from build123d import *

# Parameters (mm, degrees)
SKETCH1_W                      = 7
SKETCH1_H                      = 26.5
SKETCH2_R                      = 12.5
SHAFT_THRU_DEPTH               = 52.39066063
CBORE_FOR_M5_SHCS1_D           = 5.5
CBORE_FOR_M5_SHCS1_CBORE_D     = 10
CBORE_FOR_M5_SHCS1_CBORE_DEPTH = 5
CIRPATTERN1_COUNT              = 4
SKETCH5_R                      = 14.25
SEAL_SEAT_DEPTH                = 3.9624


with BuildPart() as part:
    # Sketch1 → Main_body (revolve)
    with BuildSketch(Plane(origin=(0, 0, 0), x_dir=(0, 0, -1), z_dir=(1, 0, 0)), mode=Mode.PRIVATE) as main_body_sk:
        with Locations((-139.159, -22.75)):
            Rectangle(SKETCH1_W, SKETCH1_H)
        with Locations((-139.159, 22.75)):
            Rectangle(SKETCH1_W, SKETCH1_H)
    revolve(main_body_sk.sketch.rotate(Axis((0, 0, 1000), (0, 0, -1)), 270), axis=Axis((0, 0, 1000), (0, 0, -1)))

    # Sketch2 → Shaft_thru (cut, through all)
    with BuildSketch(Plane(origin=(0, 0, 135.659), x_dir=(-1, 0, 0), z_dir=(0, 0, -1))):
        Circle(SKETCH2_R)
    extrude(amount=-SHAFT_THRU_DEPTH, mode=Mode.SUBTRACT)

    # CBORE for M5 SHCS1 (through all)
    with Locations(Plane.XY.offset(142.659)):
        with Locations((0, 29.3156)):
            cbore_for_m5_shcs1 = CounterBoreHole(CBORE_FOR_M5_SHCS1_D / 2, CBORE_FOR_M5_SHCS1_CBORE_D / 2, CBORE_FOR_M5_SHCS1_CBORE_DEPTH)

    # CirPattern1: CBORE for M5 SHCS1 ×4 about axis
    cirpattern1_axis = Axis((0, 0, 0), (0, 0, 1))
    for i in range(1, CIRPATTERN1_COUNT):
        add(cbore_for_m5_shcs1.rotate(cirpattern1_axis, i * 360 / CIRPATTERN1_COUNT), mode=Mode.SUBTRACT)

    # Sketch5 → seal_seat (cut)
    with BuildSketch(Plane.XY.offset(142.659)):
        Circle(SKETCH5_R)
    extrude(amount=-SEAL_SEAT_DEPTH, mode=Mode.SUBTRACT)


solid = part.part
Geometry: final body of the model. Coordinates: model frame, mm. A direction names the side the tool comes from. Coordinates: 2 decimals unless noted, no trailing zeros. Order: outer loops, then holes, each group sorted by start corner. A loop starts at its lowest first (then second) coordinate and runs counter-clockwise, first axis right, second up.
(1) Draft query along Y for faces 3 (the face through (-34.34, 10.81, 139.11)), 4 (the face through (0.6, 26.63, 136.64)), 5 (the face through (-1, -15, 142.659)), 6 (the face through (-27, 2, 137.659)). Return one class per face: pulls with the +Y half, pulls with the -Y half, needs draft (parallel to the pull), parting line crosses it, or undercut.
(2) Material intervals for probe 1 along Y at (x, z) = (0, 141.4); probe 2 along Y at (x, z) = (0, 136.6); probe 3 along X at (y, z) = (4, 140.5), sorted ascending.
(3) Section query A-A (x = 0). Return the cut outline in (y, z).
(4) Section query D-D (x = -22). Return the cut outline in (y, z), plus the area to 3 significant figures.
(5) First-contact query: pin 1 (1.5 mm diameter, centred on x = -15, z = 139, fed in from -Y); pin 2 (14 mm diameter, centred on x = 0.5, y = 5, fed in from +Z); pin 3 (4 mm diameter, centred on y = 5.5, z = 138, fed in from +X); pin 4 (1 mm diameter, centred on x = -18, z = 138.5, fed in from -Y). Flat tips, straight axial feed; report the tip coordinate or a pass-through.
(6) Section query C-C (z = 141.75). Return the cut outline in (x, y).
(7) Access query for faces 1 (the face through (27, -2, 137.659)), 2 (the face through (-0.6, -26.63, 136.64)). Directions: +Z, -Z, +X, -X, +Y, -Y. A direction counts if a zero-diameter tool reaches every point of the face in a straight line with its end or side. Return the directions, or none.
Solution:
1. face 3: parting line crosses it
1. face 4: undercut
1. face 5: needs draft
1. face 6: undercut
2. probe 1: y = -36 to -34.32, -24.32 to -14.25, 14.25 to 24.32, 34.32 to 36
2. probe 2: y = -36 to -32.07, -26.57 to -12.5, 12.5 to 26.57, 32.07 to 36
2. probe 3: x = -35.78 to -32.32, -26.32 to -13.68, 13.68 to 26.32, 32.32 to 35.78
3. outline: (-36, 135.66) - (-32.07, 135.66) - (-32.07, 137.66) - (-34.32, 137.66) - (-34.32, 142.66) - (-36, 142.66) - close; (-26.57, 135.66) - (-12.5, 135.66) - (-12.5, 138.7) - (-14.25, 138.7) - (-14.25, 142.66) - (-24.32, 142.66) - (-24.32, 137.66) - (-26.57, 137.66) - close; (12.5, 135.66) - (26.57, 135.66) - (26.57, 137.66) - (24.32, 137.66) - (24.32, 142.66) - (14.25, 142.66) - (14.25, 138.7) - (12.5, 138.7) - close; (32.07, 135.66) - (36, 135.66) - (36, 142.66) - (34.32, 142.66) - (34.32, 137.66) - (32.07, 137.66) - close
4. outline: (-28.5, 135.66) - (28.5, 135.66) - (28.5, 142.66) - (-28.5, 142.66) - close
4. area: 399 mm2
5. pin 1: stops at y = -33.06
5. pin 2: passes through
5. pin 3: stops at x = 35.83
5. pin 4: stops at y = -31.46
6. outline: circle Ø72 at (0, 0); hole circle Ø10 at (-29.32, 0); hole circle Ø28.5 at (0, 0); hole circle Ø10 at (0, -29.32); hole circle Ø10 at (0, 29.32); hole circle Ø10 at (29.32, 0)
7. face 1: +Z
7. face 2: +Z, -Z
